Autodesk Inventor part; units mm, degrees
ref_plane "YZ Plane" through (0, 0, 0) normal (1, 0, 0) x (0, 1, 0)
ref_plane "XZ Plane" through (0, 0, 0) normal (0, 1, 0) x (-1, 0, 0)
ref_plane "XY Plane" through (0, 0, 0) normal (0, 0, 1) x (1, 0, 0)
sketch "Sketch1" plane through (0, 0, 0) normal (1, 0, 0) x (0, 1, 0)
  circle A0 centre (0, 0) radius 50.8 construction
  circle A1 centre (82.55, 0) radius 31.75 construction
  circle A2 centre (-82.55, 0) radius 31.75 construction
  circle A3 centre (0, 0) radius 114.3 construction
  circle A4 centre (0, 0) radius 38.1 construction
  arc A5 (38.1, 0) -> (114.3, 0) centre (76.2, 0) ccw construction
  arc A6 (-38.1, 0) -> (139.7, 0) centre (50.8, 0) ccw construction
  line L0 (50.8, -88.9) -> (139.7, -88.9) construction
  line L1 (139.7, -88.9) -> (139.7, 0) construction
  line L2 (139.7, 0) -> (-101.6, 0) construction
  line L3 (-101.6, 0) -> (-101.6, 139.7) construction
  line L4 (-101.6, 139.7) -> (139.7, 139.7) construction
  line L5 (139.7, 139.7) -> (139.7, 0) construction
  arc A7 (11.0716, 139.7) -> (-101.6, 96.52) centre (0, 0) ccw construction
  line L6 (-101.6, 139.7) -> (-101.6, 63.1817) construction
  line L7 (-101.6, 63.1817) -> (-95.25, 63.1817) construction
  arc A8 (-11.0716, 139.7) -> (-101.6, 96.52) centre (0, 0) ccw
  line L8 (-11.0716, 139.7) -> (139.7, 139.7)
  line L9 (139.7, 139.7) -> (139.7, -88.9)
  line L10 (139.7, -88.9) -> (50.8, -88.9)
  arc A9 (-38.1, 0) -> (50.8, -88.9) centre (50.8, 0) ccw
  arc A10 (38.1, 0) -> (-38.1, 0) centre (0, 0) ccw
  arc A11 (38.1, 0) -> (114.3, 0) centre (76.2, 0) ccw
  arc A12 (114.3, 0) -> (-95.25, 63.1817) centre (0, 0) ccw
  line L11 (-95.25, 63.1817) -> (-101.6, 63.1817)
  line L12 (-101.6, 96.52) -> (-101.6, 63.1817)
  dimension "d1" = 63.5
  dimension "d0" = 101.6
  dimension "d2" = 63.5
  dimension "d3" = 82.55
  dimension "d4" = 82.55
  dimension "d5" = 0
  dimension "d6" = 0
  dimension "d7" = 228.6
  dimension "d8" = 76.2
  dimension "d9" = 76.2
  dimension "d10" = 177.8
  dimension "d11" = 88.9
  dimension "d12" = 139.7
  dimension "d13" = 0
  dimension "d14" = 241.3
  dimension "d15" = 139.7
  dimension "d16" = 0
  dimension "d76" = 6.35
  dimension "d77" = 43.18
extrude "Extrusion1" add sketch "Sketch1" along normal blind 3.175
sketch "Sketch2" plane through (3.175, 0, 0) normal (1, 0, 0) x (0, 0, -1)
  arc A0 (0, 38.1) -> (0, -38.1) centre (0, 0) ccw
  arc A1 (0, -38.1) -> (88.9, 50.8) centre (0, 50.8) ccw
  line L0 (88.9, 50.8) -> (88.9, 139.7)
  line L1 (88.9, 139.7) -> (-139.7, 139.7)
  line L2 (-139.7, 139.7) -> (-139.7, -11.0716)
  arc A2 (-139.7, -11.0716) -> (-96.52, -101.6) centre (0, 0) ccw
  line L3 (-96.52, -101.6) -> (-63.1817, -101.6)
  line L4 (-63.1817, -101.6) -> (-63.1817, -95.25)
  arc A3 (0, 114.3) -> (-63.1817, -95.25) centre (0, 0) ccw
  arc A4 (0, 38.1) -> (0, 114.3) centre (0, 76.2) ccw
  line L5 (-63.1817, -101.6) -> (-139.3817, -101.6)
  line L6 (-139.3817, -101.6) -> (-139.3817, -95.25)
  line L7 (-139.3817, -95.25) -> (-63.1817, -95.25)
  line L8 (-63.1817, -95.25) -> (-63.1817, -101.6)
  arc A5 (0, 114.3) -> (-63.1817, -95.25) centre (0, 0) ccw
  line L9 (-63.1817, -101.6) -> (-71.842, -101.6)
  line L10 (-71.842, -101.6) -> (-71.842, -88.9)
  line L11 (-71.842, -88.9) -> (-63.1817, -88.9)
  line L12 (-63.1817, -88.9) -> (-63.1817, -101.6)
  point P0 (0, 0)
  dimension "d24" = 76.2
  dimension "d25" = 6.35
  dimension "d26" = 12.7
extrude "Extrusion2" cut sketch "Sketch2" against normal blind 3.175 contours L11 L12 A3 | A3 L7 L10 | L4 L3 L10 L7 | L10 L3 A2 L7 | A2 L5 L6 L7
sketch "Sketch3" plane through (3.175, 0, 0) normal (1, 0, 0) x (0, 0, -1)
  line L0 (-102.7916, -95.25) -> (-71.842, -95.25)
  line L1 (-71.842, -95.25) -> (-71.842, -88.9)
  arc A0 (0, 114.3) -> (-71.842, -88.9) centre (0, 0) ccw
  arc A1 (0, 38.1) -> (0, 114.3) centre (0, 76.2) ccw
  arc A2 (0, 38.1) -> (0, -38.1) centre (0, 0) ccw
  arc A3 (0, -38.1) -> (88.9, 50.8) centre (0, 50.8) ccw
  line L2 (88.9, 50.8) -> (88.9, 139.7)
  line L3 (88.9, 139.7) -> (-139.7, 139.7)
  line L4 (-139.7, 139.7) -> (-139.7, -11.0716)
  arc A4 (-139.7, -11.0716) -> (-102.7916, -95.25) centre (0, 0) ccw
  point P0 (0, 0)
  point P1 (-127, 127)
  point P2 (76.2, 127)
  point P3 (-95.25, -82.55)
  point P4 (-127, 0)
  dimension "d29" = 12.7
  dimension "d30" = 12.7
  dimension "d31" = 12.7
  dimension "d32" = 12.7
  dimension "d33" = 12.7
  dimension "d34" = 139.7
  dimension "d35" = 95.25
  dimension "d36" = 82.55
hole "Hole1" at (3.175, 127, 127) at (3.175, 127, -76.2) at (3.175, -82.55, 95.25) at (3.175, 0, 127) direction (-1, 0, 0) diameter 6.35 end through all
sketch "Sketch4" plane through (3.175, 0, 0) normal (1, 0, 0) x (0, 0, -1)
  circle A0 centre (-95.25, -82.55) radius 3.175
  circle A1 centre (-127, 127) radius 3.175
  circle A2 centre (76.2, 127) radius 3.175
  circle A3 centre (-127, 0) radius 3.175
  line L0 (-102.7916, -95.25) -> (-71.842, -95.25)
  line L1 (-71.842, -95.25) -> (-71.842, -88.9)
  arc A4 (0, 114.3) -> (-71.842, -88.9) centre (0, 0) ccw
  arc A5 (0, 38.1) -> (0, 114.3) centre (0, 76.2) ccw
  arc A6 (0, 38.1) -> (0, -38.1) centre (0, 0) ccw
  arc A7 (0, -38.1) -> (88.9, 50.8) centre (0, 50.8) ccw
  line L2 (88.9, 50.8) -> (88.9, 139.7)
  line L3 (88.9, 139.7) -> (-139.7, 139.7)
  line L4 (-139.7, 139.7) -> (-139.7, -11.0716)
  arc A8 (-139.7, -11.0716) -> (-102.7916, -95.25) centre (0, 0) ccw
  circle A9 centre (0, 0) radius 3.175
  point P0 (0, 0)
  dimension "d55" = 6.35
sketch "Sketch5" plane through (3.175, 0, 0) normal (1, 0, 0) x (0, 0, -1)
  circle A0 centre (-95.25, -82.55) radius 3.175
  circle A1 centre (-127, 127) radius 3.175
  circle A2 centre (76.2, 127) radius 3.175
  circle A3 centre (-127, 0) radius 3.175
  line L0 (-102.7916, -95.25) -> (-71.842, -95.25)
  line L1 (-71.842, -95.25) -> (-71.842, -88.9)
  arc A4 (0, 114.3) -> (-71.842, -88.9) centre (0, 0) ccw
  arc A5 (0, 38.1) -> (0, 114.3) centre (0, 76.2) ccw
  arc A6 (0, 38.1) -> (0, -38.1) centre (0, 0) ccw
  arc A7 (0, -38.1) -> (88.9, 50.8) centre (0, 50.8) ccw
  line L2 (88.9, 50.8) -> (88.9, 139.7)
  line L3 (88.9, 139.7) -> (-139.7, 139.7)
  line L4 (-139.7, 139.7) -> (-139.7, -11.0716)
  arc A8 (-139.7, -11.0716) -> (-102.7916, -95.25) centre (0, 0) ccw
  line L5 (-139.7, -11.0716) -> (-139.7, -95.25) construction
  line L6 (-139.7, -95.25) -> (-102.7916, -95.25) construction
  line L7 (-139.7, -95.25) -> (-127, -95.25) construction
  line L8 (-127, -95.25) -> (-127, -82.55) construction
  line L9 (-127, -82.55) -> (-139.7, -82.55) construction
  line L10 (-139.7, -82.55) -> (-139.7, -95.25) construction
  line L11 (-139.7, -11.0716) -> (-139.7, -82.55)
  line L12 (-139.7, -82.55) -> (-127, -95.25)
  line L13 (-127, -95.25) -> (-102.7916, -95.25)
  point P0 (0, 0)
  dimension "d60" = 12.7
  dimension "d61" = 12.7
extrude "Extrusion4" add sketch "Sketch5" against normal blind 3.175 contours L13 L12 L11 A8
sketch "Sketch6" plane through (3.175, 0, 0) normal (1, 0, 0) x (0, 0, -1)
  circle A0 centre (-95.25, -82.55) radius 3.175
  circle A1 centre (-127, 127) radius 3.175
  circle A2 centre (76.2, 127) radius 3.175
  circle A3 centre (-127, 0) radius 3.175
  line L0 (-127, -95.25) -> (-71.842, -95.25)
  line L1 (-71.842, -95.25) -> (-71.842, -88.9)
  arc A4 (0, 114.3) -> (-71.842, -88.9) centre (0, 0) ccw
  arc A5 (0, 38.1) -> (0, 114.3) centre (0, 76.2) ccw
  arc A6 (0, 38.1) -> (0, -38.1) centre (0, 0) ccw
  arc A7 (0, -38.1) -> (88.9, 50.8) centre (0, 50.8) ccw
  line L2 (88.9, 50.8) -> (88.9, 139.7)
  line L3 (88.9, 139.7) -> (-139.7, 139.7)
  line L4 (-139.7, 139.7) -> (-139.7, -82.55)
  line L5 (-139.7, -82.55) -> (-127, -95.25)
  point P0 (0, 0)
  point P1 (-123.825, -85.725)
  dimension "d64" = 15.875
  dimension "d65" = 9.525
hole "Hole3" at (3.175, -85.725, 123.825) direction (-1, 0, 0) diameter 9.525 end through all
fillet "Fillet1" radius 3.175 2 edges at (1.5875, -95.25, 71.842) (1.5875, -88.9, 71.842)
extrude "Extrusion5" cut sketch "Sketch4" against normal blind 25.4 contours A9
properties part number "rail" material "Aluminum 6061"
Geometry: final body of the model. Coordinates: model frame, mm. A direction names the side the tool comes from. Give positions to 0.01 mm unless a question says otherwise; leave off trailing zeros. Loops run counter-clockwise (first coordinate to the right, second up) from the corner with the lowest first, then second, coordinate; pieces in that order, holes last. Notation, with made-up numbers: (31.25, -10.75) -> (57.25, -10.75) arc R6 ccw to (57.25, -3.75) -> close; hole circle Ø3 at (21.25, 88). An arc over 180 degrees is marked (long way). Return JSON: item names as keys, results as strings.
Item 1: Pin query (flat end, axial travel): P1, Ø5.5, axis at y = -85.725, z = 123.825, coming from the +X side; P2, Ø0.8, axis at x = 1.5, y = -91.5, coming from the -Z side; P3, Ø1.5, axis at x = 2, y = -14.5, coming from the -Z side. Return the tip coordinate at first contact, or that it passes through.
Filled in:
{"P1": "through", "P2": "z = 71.84", "P3": "z = -61.13"}
Item 2: Section A-A, the plane y = 127. Output: boundary loops of the cut face in (x, z) (3 decimals), plus the area to 3 significant figures.
Filled in:
{"outline": "(0, -88.9) -> (3.175, -88.9) -> (3.175, -79.375) -> (0, -79.375) -> close; (0, -73.025) -> (3.175, -73.025) -> (3.175, 123.825) -> (0, 123.825) -> close; (0, 130.175) -> (3.175, 130.175) -> (3.175, 139.7) -> (0, 139.7) -> close", "area": "685 mm^2"}
Item 3: Section C-C, the plane x = 2.3. Count the separate pieces of the cut face and the enclosed holes in it, plus the area to 3 significant figures.
Filled in:
{"separate pieces": "1", "enclosed holes": "6", "area": "26,900 mm^2"}
Item 4: Section B-B, the plane z = 102. Output: boundary loops of the cut face in (x, y) (3 decimals), plus the area to 3 significant figures.
Filled in:
{"outline": "(0, -95.25) -> (3.175, -95.25) -> (3.175, -51.58) -> (0, -51.58) -> close; (0, 51.58) -> (3.175, 51.58) -> (3.175, 139.7) -> (0, 139.7) -> close", "area": "418 mm^2"}
Item 5: Access query for faces 4 (the cylindrical face through (1.565, 36.95, 108.163)), 5 (the flat face through (3.175, 24, 27)). Directions: +Z, -Z, +X, -X, +Y, -Y. A direction counts if a zero-diameter tool reaches every point of the face in a straight line with its end or side. Return the directions, or none.
Filled in:
{"face 4": "+X, -X", "face 5": "+Z, -Z, +X, +Y, -Y"}
Item 6: Line query: line 1 (Z direction, x = 0.75, y = 126.5); line 2 (Y direction, x = 1.6, z = 127) (3 decimals); line 3 (Y direction, x = 0.2, z = -77). Output: solid intervals per line, ascending.
Filled in:
{"line 1": "-88.9 to -79.34, -73.06 to 123.86, 130.14 to 139.7", "line 2": "-95.25 to -89.275, -82.175 to -3.175, 3.175 to 123.825, 130.175 to 139.7", "line 3": "6.37 to 123.93, 130.07 to 139.7"}
Item 7: Section D-D, the plane y = 22.5. Output: boundary loops of the cut face in (x, z) (3 decimals).
Filled in:
{"outline": "(0, -84.275) -> (3.175, -84.275) -> (3.175, 30.747) -> (0, 30.747) -> close; (0, 112.064) -> (3.175, 112.064) -> (3.175, 139.7) -> (0, 139.7) -> close"}
Item 8: Mould query, pull axis Y, two halves, no side actions, for faces 1 (the flat face through (0, 24, 27)), 2 (the cylindrical face through (1.565, -87.156, 119.282)), 3 (the cylindrical face through (1.565, -11.367, -63.549)). Classes: released by +Y, released by -Y, zero draft, split by the parting line, or undercut.
Filled in:
{"face 1": "zero draft", "face 2": "undercut", "face 3": "released by -Y"}
